from build123d import *

# Parameters (mm, degrees)
F1_DEPTH = 76.2
F3_R     = 4.699
F4_DEPTH = 19.05
F5_DEPTH = 26.162


with BuildPart() as f1:
    # F0 (on Right) → F1 (new body)
    with BuildSketch(Plane.YZ):
        Polygon((-50.8, -31.816228), (44.45, -31.816228), (44.45, -12.766228), (0, -12.766228), (0, 38.033772), (-25.4, 38.033772), (-25.4, -12.766228), (-50.8, -12.766228), align=None)
    extrude(amount=F1_DEPTH)

    # F3 (on face) → F4 (cut)
    with BuildSketch(Plane.XY.offset(-12.766228)):
        with Locations((63.56959, 31.471644)):
            Circle(F3_R)
        with Locations((12.7, 31.471644)):
            Circle(F3_R)
        with Locations((12.7, -38.98726)):
            Circle(F3_R)
        with Locations((63.881002, -38.98726)):
            Circle(F3_R)
    extrude(amount=-F4_DEPTH, mode=Mode.SUBTRACT)

    # F2 (on Front) → F5 (cut)
    with BuildSketch(Plane.XZ):
        Polygon((51.643919, 9.441765), (51.643919, 38.016765), (23.8252, 38.07896), (23.8252, 9.50396), align=None)
    extrude(amount=F5_DEPTH, mode=Mode.SUBTRACT)


solid = f1.part
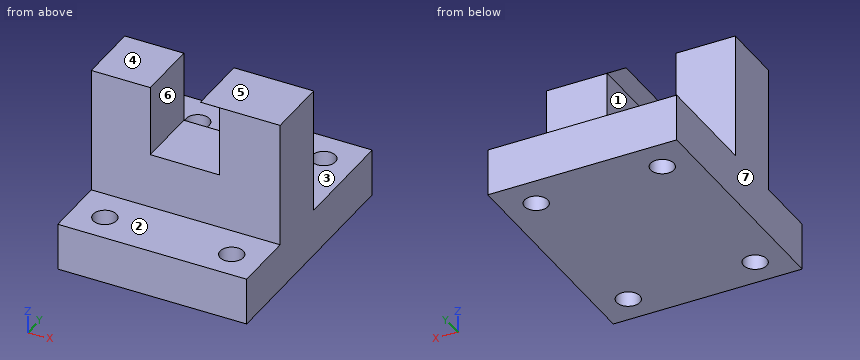
Could you check a few things on this model? Use its own coordinates, in mm. Face numbers are marked on the shaded views. A direction names the side the tool comes from. Round coordinates to 2 decimals unless told otherwise and drop trailing zeros. Write each loop counter-clockwise with the first axis right and the second up, starting at its lowest first coordinate (ties: lowest second). Pieces come first, ordered by that corner, then holes. Notation, with made-up numbers: (34.25, 18) - (54.25, 18) arc R21 cw to (54.25, 29) - close; hole circle Ø4 at (41, 88.5). An arc over 180 degrees is marked (long way). Put each result on its own line as item: value. Start each with the question number.
(1) I want a section at D-D, the plane z = -18. Please give me the cut outline in (x, y).
(2) For the marked faces 1, 2, 3 and 4, which set-ups out of +Z, -Z, +X, -X, +Y, -Y let a thin tool reach every point of the face, with its end or its side?
(3) Thinking about a two-plate mould opening in X: for the marked faces 5, 6 and 7, which applies, released by +X, released by -X, zero draft, split by the parting line, or undercut?
(4) I need wall thicknesses on probe 1 along Y at (x, z) = (12.7, -21); probe 2 along X at (y, z) = (33, -16.5); probe 3 along X at (y, z) = (-18.5, 14.5). Which ranges of each line are inside material? Lowest first, please.
(5) I want a section at A-A, the plane z = 28. Please give me the cut outline in (x, y).
(6) I want a section at C-C, the plane y = -3. Please give me the cut outline in (x, z).
(7) Will these pins go through, and if not, where does the flat tip stop? pin 1 (1.5 mm diameter, centred on x = 56, z = 20, fed in from +Y); pin 2 (12.5 mm diameter, centred on x = 55.5, y = -36, fed in from +Z); pin 3 (8 mm diameter, centred on x = 55, z = 25.5, fed in from -Y).
(8) I want a section at B-B, the plane x = 12.7. Please give me the cut outline in (y, z), plus the area to 3 significant figures.
Here are the results:
1. outline: (0, -50.8) - (76.2, -50.8) - (76.2, 44.45) - (0, 44.45) - close; hole circle Ø9.4 at (12.7, -38.99); hole circle Ø9.4 at (12.7, 31.47); hole circle Ø9.4 at (63.57, 31.47); hole circle Ø9.4 at (63.88, -38.99)
2. face 1: +Y, -Y
2. face 2: +Z, +X, -X, -Y
2. face 3: +Z, +X, -X, +Y
2. face 4: +Z, +X, -X, +Y, -Y
3. face 5: zero draft
3. face 6: undercut
3. face 7: released by -X
4. probe 1: y = -50.8 to -43.69, -34.29 to 26.77, 36.17 to 44.45
4. probe 2: x = 0 to 8.26, 17.14 to 59.13, 68.01 to 76.2
4. probe 3: x = 0 to 23.83, 51.64 to 76.2
5. outline: (0, -25.4) - (23.83, -25.4) - (23.83, 0) - (0, 0) - close; (51.64, -25.4) - (76.2, -25.4) - (76.2, 0) - (51.64, 0) - close
6. outline: (0, -31.82) - (76.2, -31.82) - (76.2, 38.03) - (44.04, 38.03) - (51.64, 38.02) - (51.64, 9.44) - (23.83, 9.5) - (23.83, 38.03) - (0, 38.03) - close
7. pin 1: stops at y = 0
7. pin 2: stops at z = -12.77
7. pin 3: stops at y = -25.4
8. outline: (-50.8, -31.82) - (-43.69, -31.82) - (-43.69, -12.77) - (-50.8, -12.77) - close; (-34.29, -31.82) - (26.77, -31.82) - (26.77, -12.77) - (0, -12.77) - (0, 38.03) - (-25.4, 38.03) - (-25.4, -12.77) - (-34.29, -12.77) - close; (36.17, -31.82) - (44.45, -31.82) - (44.45, -12.77) - (36.17, -12.77) - close
8. area: 2,750 mm^2
